Check sheet for the drawn part. Datum: minimum x, y, z corner. Units: mm. A direction names the side the tool comes from. Round coordinates to 2 decimals unless told otherwise and drop trailing zeros. Write each loop counter-clockwise with the first axis right and the second up, starting at its lowest first coordinate (ties: lowest second). Pieces come first, ordered by that corner, then holes. Notation, with made-up numbers: (88.5, 77) - (108.5, 77) arc R18 ccw to (108.5, 92) - close; hole circle Ø6 at (51.5, -17.75). An arc over 180 degrees is marked (long way). Answer as a JSON object with one key per item and string values.
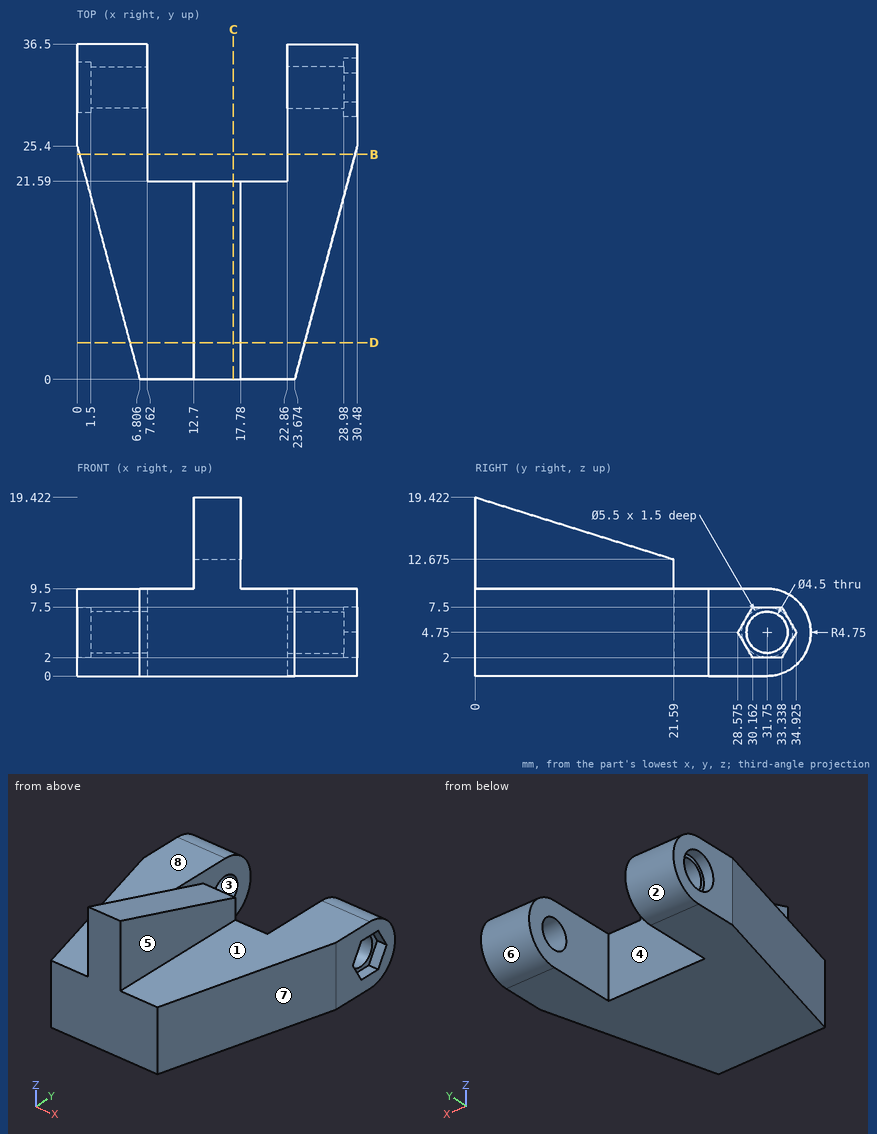
1. Cross-section at B-B (y = 24.5). Record the boundary of the cut face in (x, z), plus the area to 3 significant figures.
Completed:
{"outline": "(0.24, 0) - (7.62, 0) - (7.62, 9.5) - (0.24, 9.5) - close; (22.86, 0) - (30.24, 0) - (30.24, 9.5) - (22.86, 9.5) - close", "area": "140 mm^2"}
2. Access from +Z, -Z, +X, -X, +Y, -Y to the whole of each face (thin tool, end or side, straight path). Record for the marked faces 4, 5, 6, 7 and 8.
Completed:
{"face 4": "+Z, -Z, +Y", "face 5": "+Z, +X, +Y, -Y", "face 6": "+X, -X, +Y", "face 7": "+Z, -Z, +X, -Y", "face 8": "+Z, -X, +Y, -Y"}
3. Mould release check, pull along Z, two halves, no side actions. Record for the marked faces 1, 2 and 3: released by +Z, released by -Z, zero draft, split by the parting line, or undercut.
Completed:
{"face 1": "released by +Z", "face 2": "split by the parting line", "face 3": "undercut"}
4. Cross-section at D-D (y = 4). Record the boundary of the cut face in (x, z).
Completed:
{"outline": "(5.73, 0) - (24.75, 0) - (24.75, 9.5) - (17.78, 9.5) - (17.78, 18.17) - (12.7, 18.17) - (12.7, 9.5) - (5.73, 9.5) - close"}
5. Cross-section at C-C (x = 17). Record the boundary of the cut face in (y, z) (1 decimal).
Completed:
{"outline": "(0, 0) - (21.6, 0) - (21.6, 12.7) - (0, 19.4) - close"}
6. Go/stop test with flat-tipped pins: pin 1 (10 mm diameter, centred on x = 10.5, y = 10.5, fed in from +Z); pin 2 (6 mm diameter, centred on x = 6, y = 20.5, fed in from +Z); pin 3 (6 mm diameter, centred on y = 17, z = 13.5, fed in from +X). Record where each tip stops, or that it passes through.
Completed:
{"pin 1": "stops at z = 17.54", "pin 2": "stops at z = 9.5", "pin 3": "stops at x = 17.78"}
7. Material ranges on probe 1 along X at (y, z) = (29, 7.25); probe 2 along Z at (x, y) = (24.5, 6.5); probe 3 along Y at (x, z) = (9, 3.5), recorded low to high. Write a range as from..to.
Completed:
{"probe 1": "x = 0..7.62, 22.86..30.48", "probe 2": "z = 0..9.5", "probe 3": "y = 0..21.59"}
